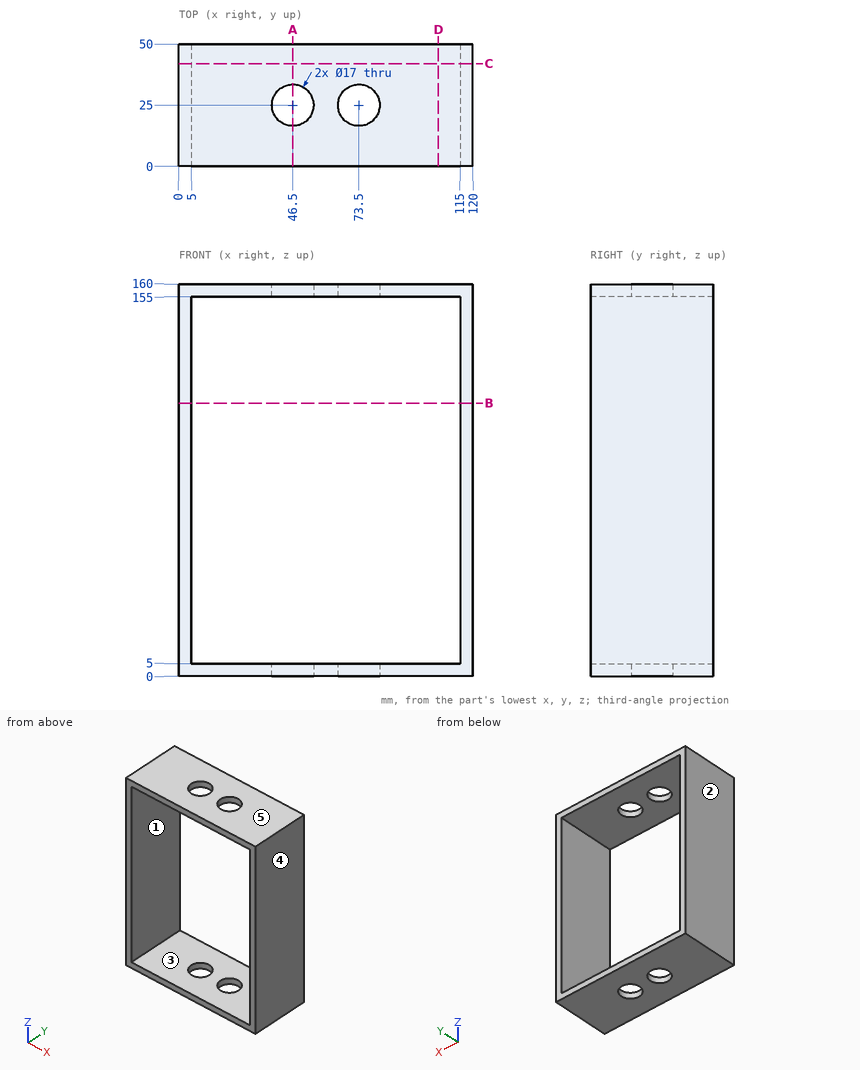
Part print with two shaded views. Sizes in mm from the minimum x, y, z corner. A direction names the side the tool comes from. Round coordinates to 2 decimals unless told otherwise and drop trailing zeros. Order: outer loops, then holes, each group sorted by start corner. A loop starts at its lowest first (then second) coordinate and runs counter-clockwise, first axis right, second up. Notation, with made-up numbers: (2, 40) - (41, 40) arc R20 ccw to (41, 51) - close; hole circle Ø7 at (-38, 19.25). An arc over 180 degrees is marked (long way). Answer in a Markdown table with one row per item. Add a question column.
(1) Band-saw the part on C-C on y = 42. List the corners of the cut face in (x, z).
(2) 3-axis set-ups, long thin cutter, end or side, ignore diameter. For the marked faces 1 and 2: which of +Z, -Z, +X, -X, +Y, -Y reach the whole face in a straight line?
(3) Drop a flat-ended pin along its axis: pin 1 Ø5 at (x, y) = (105.5, 34.5) entering from -Z. Give the stop position or say it passes through.
(4) Band-saw the part on D-D on x = 106. List the corners of the cut face in (y, z), and give its area (3 significant figures).
(5) Probe L1, parallel to Y at x = 46, z = 2; L2, parallel to X at y = 16.5, z = 52.5; L3, parallel to Z at x = 8, y = 17.5. List the from-to ranges inside material, lowest first. Write a range as [from, to].
(6) Band-saw the part on B-B on z = 111.5. List the corners of the cut face in (x, y), and give its area (3 significant figures).
(7) Band-saw the part on A-A on x = 46.5. List the corners of the cut face in (y, z).
(8) Mould opens along Z. For the marked faces 3, 4 and 5 say: +Z half, -Z half, draft (parallel to the pull), parting line (faces both ways), or undercut.
Data:
| question | item | result |
|---|---|---|
| 1 | outline | (0, 0) - (120, 0) - (120, 160) - (0, 160) - close; hole (5, 5) - (115, 5) - (115, 155) - (5, 155) - close |
| 2 | face 1 | +Y, -Y |
| 2 | face 2 | +Z, -Z, -X, +Y, -Y |
| 3 | pin 1 | stops at z = 0 |
| 4 | outline | (0, 0) - (50, 0) - (50, 5) - (0, 5) - close; (0, 155) - (50, 155) - (50, 160) - (0, 160) - close |
| 4 | area | 500 mm^2 |
| 5 | L1 | y = [0, 16.51], [33.49, 50] |
| 5 | L2 | x = [0, 5], [115, 120] |
| 5 | L3 | z = [0, 5], [155, 160] |
| 6 | outline | (0, 0) - (5, 0) - (5, 50) - (0, 50) - close; (115, 0) - (120, 0) - (120, 50) - (115, 50) - close |
| 6 | area | 500 mm^2 |
| 7 | outline | (0, 0) - (16.5, 0) - (16.5, 5) - (0, 5) - close; (0, 155) - (16.5, 155) - (16.5, 160) - (0, 160) - close; (33.5, 0) - (50, 0) - (50, 5) - (33.5, 5) - close; (33.5, 155) - (50, 155) - (50, 160) - (33.5, 160) - close |
| 8 | face 3 | undercut |
| 8 | face 4 | draft |
| 8 | face 5 | +Z half |
